Here's how the part is built. I have some questions about the finished solid (model axes, mm). A direction names the side the tool comes from. Give positions to 0.01 mm unless a question says otherwise; leave off trailing zeros. Loops run counter-clockwise (first coordinate to the right, second up) from the corner with the lowest first, then second, coordinate; pieces in that order, holes last.
Q1. I need wall thicknesses on line 1 (X direction, y = 1.4, z = -25); line 2 (Z direction, x = 10, y = 1.1); line 3 (Y direction, x = 20, z = 0.65). Which ranges of each line are inside material? Lowest first, please.
Q2. We'd pull the mould along X, two halves only. Please class faces 4 (the face through (55, 14, 1)), 5 (the face through (27, 1, -43)), 6 (the face through (0, 14, 1)), 7 (the face through (42, 1, -25)): +X half, -X half, draft (parallel to the pull), parting line (faces both ways), or undercut.
Q3. If we section it at B-B (z = -25): Please give me the cut outline in (x, y), plus the area to 3 significant figures.
Q4. If we section it at C-C (y = 41.5): Please give me the cut outline in (x, z), plus the area to 3 significant figures.
Q5. For faces 1 (the face through (38, 35, 1)), 2 (the face through (28, 2, -21)), 3 (the face through (27, 25, 2)), which set-ups out of +Z, -Z, +X, -X, +Y, -Y let a thin tool reach every point of the face, with its end or its side?
Q6. If we section it at A-A (x = 20): Please give me the cut outline in (y, z), plus the area to 3 significant figures.
Q7. Will these pins go through, and if not, where does the flat tip stop? P1, Ø12, axis at x = 33.5, y = 15.5, coming from the -Z side; P2, Ø8, axis at x = 5.5, z = -30, coming from the -Y side; P3, Ø5, axis at x = 29, z = -10, coming from the +Y side.
Q8. If we section it at D-D (x = 10): Please give me the cut outline in (y, z), plus the area to 3 significant figures.
Autodesk Inventor part; units mm, degrees
ref_plane "YZ Plane" through (0, 0, 0) normal (1, 0, 0) x (0, 1, 0)
ref_plane "XZ Plane" through (0, 0, 0) normal (0, 1, 0) x (-1, 0, 0)
ref_plane "XY Plane" through (0, 0, 0) normal (0, 0, 1) x (1, 0, 0)
sketch "Sketch1" plane through (0, 0, 0) normal (0, 0, 1) x (1, 0, 0)
  line L0 (0, 0) -> (55, 0)
  line L1 (55, 0) -> (55, 50)
  line L2 (55, 50) -> (0, 50)
  line L3 (0, 50) -> (0, 0)
  dimension "d3" = 55
  dimension "d4" = 50
extrude "Extrusion1" add sketch "Sketch1" along normal blind 2
sketch "Sketch2" plane through (0, 0, 2) normal (0, 0, 1) x (1, 0, 0)
  circle A0 centre (20, 35) radius 8
  line L0 (0, 0) -> (55, 0)
  line L1 (0, 50) -> (0, 0)
  line L2 (35, 37) -> (38, 37)
  line L3 (38, 37) -> (38, 33)
  line L4 (38, 33) -> (35, 33)
  line L5 (35, 33) -> (35, 37)
  dimension "d2" = 16
  dimension "d5" = 35
  dimension "d6" = 20
  dimension "d7" = 15
  dimension "d8" = 4
  dimension "d9" = 3
  dimension "d10" = 2
extrude "Extrusion2" cut sketch "Sketch2" against normal through all
sketch "Sketch4" plane through (0, 0, 2) normal (0, 0, 1) x (1, 0, 0)
  line L0 (0, 2) -> (0, 0)
  line L1 (0, 0) -> (55, 0)
  line L2 (55, 0) -> (55, 2)
  line L3 (55, 2) -> (0, 2)
  line L4 (0, 2) -> (0, 0)
  dimension "d26" = 2
  dimension "d27" = 55
extrude "Extrusion3" add sketch "Sketch4" against normal blind 45
sketch "Sketch6" plane through (0, 2, 0) normal (0, 1, 0) x (1, 0, 0)
  circle A0 centre (10, 25) radius 3
  circle A1 centre (45, 25) radius 3
  line L0 (0, 0) -> (0, 43)
  line L1 (55, 0) -> (55, 43)
  line L2 (0, 43) -> (55, 43)
  dimension "d28" = 6
  dimension "d29" = 6
  dimension "d30" = 10
  dimension "d31" = 10
  dimension "d32" = 18
  dimension "d33" = 18
extrude "Extrusion5" cut sketch "Sketch6" against normal through all
properties part number "POT mount" material "Nylon 6/6"
Check sheet entries:
1. line 1: x = 0 to 7, 13 to 42, 48 to 55
1. line 2: z = -43 to -28, -22 to 2
1. line 3: y = 0 to 27, 43 to 50
2. face 4: +X half
2. face 5: draft
2. face 6: -X half
2. face 7: undercut
3. outline: (0, 0) - (7, 0) - (7, 2) - (0, 2) - close; (13, 0) - (42, 0) - (42, 2) - (13, 2) - close; (48, 0) - (55, 0) - (55, 2) - (48, 2) - close
3. area: 86.0 mm2
4. outline: (0, 0) - (15.34, 0) - (15.34, 2) - (0, 2) - close; (24.66, 0) - (55, 0) - (55, 2) - (24.66, 2) - close
4. area: 91.3 mm2
5. face 1: +Z, -Z
5. face 2: -Z, +X, -X, +Y
5. face 3: +Z, +X, -X, +Y, -Y
6. outline: (0, -43) - (2, -43) - (2, 0) - (27, 0) - (27, 2) - (0, 2) - close; (43, 0) - (50, 0) - (50, 2) - (43, 2) - close
6. area: 154 mm2
7. P1: stops at z = 0
7. P2: stops at y = 0
7. P3: stops at y = 2
8. outline: (0, -43) - (2, -43) - (2, -28) - (0, -28) - close; (0, -22) - (2, -22) - (2, 0) - (50, 0) - (50, 2) - (0, 2) - close
8. area: 174 mm2
